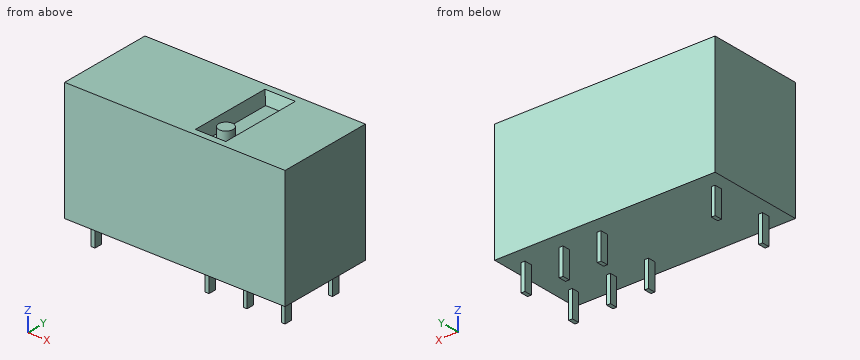
```python
from build123d import *

# Parameters (mm, degrees)
F0_W     = 12.7
F0_H     = 15.7
F1_DEPTH = 14.5
F2_W     = 0.5
F2_H     = 1
F3_DEPTH = 3.5
F4_W     = 4
F4_H     = 11
F4_R     = 0.9543570249
F5_DEPTH = 1.5
F6_SIZE2 = 1.49999
F6_SIZE  = 0.49999


# Not quite as in the source:
# - a fillet or chamfer is up to 0.001 mm smaller than in the source, because OpenCascade refuses the exact size


with BuildPart() as f1:
    # F0 (on Right) → F1 (new body, symmetric)
    with BuildSketch(Plane.YZ):
        with Locations((0, 7.85)):
            Rectangle(F0_W, F0_H)
    extrude(amount=F1_DEPTH, both=True)

    # F2 (on Top) → F3 (join)
    with BuildSketch(Plane.XY):
        with Locations((-12.5, 3.75)):
            Rectangle(F2_W, F2_H)
        with Locations((2.5, 3.75)):
            Rectangle(F2_W, F2_H)
        with Locations((7.5, 3.75)):
            Rectangle(F2_W, F2_H)
        with Locations((12.5, 3.75)):
            Rectangle(F2_W, F2_H)
        with Locations((2.5, -3.75)):
            Rectangle(F2_W, F2_H)
        with Locations((7.5, -3.75)):
            Rectangle(F2_W, F2_H)
        with Locations((12.5, -3.75)):
            Rectangle(F2_W, F2_H)
        with Locations((-12.5, -3.75)):
            Rectangle(F2_W, F2_H)
    extrude(amount=-F3_DEPTH)

    # F4 (on face) → F5 (cut)
    with BuildSketch(Plane.XY.offset(15.7)):
        with Locations((4, 0)):
            Rectangle(F4_W, F4_H)
        with Locations((4, -3.076559362)):
            Circle(F4_R, mode=Mode.SUBTRACT)
    extrude(amount=-F5_DEPTH, mode=Mode.SUBTRACT)

    # F6 (size 0.5 and 1.5 in the source; OpenCascade refuses exactly that, so slightly less here)
    f6_edges = [f1.edges().sort_by_distance(p)[0] for p in [
        (2, 0, 14.2),
        (4, 5.5, 14.2),
        (6, 0, 14.2),
        (4, -5.5, 14.2),
    ]]
    f6_side = f1.faces().sort_by_distance((4, 0.213987, 14.2))[0]
    chamfer(f6_edges, length=F6_SIZE, length2=F6_SIZE2, reference=f6_side)


solid = f1.part
```
The model under review builds one solid part; all positions refer to its coordinate system, in mm. Coordinates: 2 decimals unless noted, no trailing zeros. Write each loop counter-clockwise with the first axis right and the second up, starting at its lowest first coordinate (ties: lowest second). Pieces come first, ordered by that corner, then holes. Notation, with made-up numbers: (9.5, 43.5) - (52.5, 43.5) arc R25 ccw to (52.5, 74.5) - close; hole circle Ø9 at (-22, -32.75). An arc over 180 degrees is marked (long way). Answer in a Markdown table with one row per item. Add a question column.
Q1. To check wall thickness, follow line 1 along Z through (x, y) = (11.5, -5.5). State the ranges of the line that lie inside material, in increasing order. Write a range as from..to.
Q2. Clearance check with flat-ended pins moving along their axes: pin 1 (1.1 mm diameter, centred on y = -4, z = -2.5, fed in from +X); pin 2 (0.9 mm diameter, centred on x = 3.5, y = 1, fed in from +Z); pin 3 (1.1 mm diameter, centred on y = 3.5, z = -2, fed in from -X). State where each tip first meets the part, or that it passes through.
Q3. Consider section C-C on x = 11.5. Give the boundary of the cut face in (y, z), then the cut area to 3 significant figures.
Answers below:
| question | item | result |
|---|---|---|
| 1 | line 1 | 0..15.7 |
| 2 | pin 1 | x = 12.75 |
| 2 | pin 2 | z = 14.2 |
| 2 | pin 3 | x = -12.75 |
| 3 | outline | (-6.35, 0) - (6.35, 0) - (6.35, 15.7) - (-6.35, 15.7) - close |
| 3 | area | 199 mm² |
